from build123d import *

# Parameters (mm, degrees)
SKETCH1_W                      = 85
SKETCH1_H                      = 90
BOSS_EXTRUDE1_BASE_DEPTH       = 3
BOSS_EXTRUDE4_SIDE_WALLS_DEPTH = 90
CUT_EXTRUDE2_GUIDE_HOLES_DEPTH = 133.830719339
SKETCH15_W                     = 85
SKETCH15_H                     = 20
BOSS_EXTRUDE9_REAR_WALL_DEPTH  = 3
BOSS_EXTRUDE1_START            = 3
SKETCH17_W                     = 85
SKETCH17_H                     = 3
BOSS_EXTRUDE1_REAR_WALL_DEPTH  = 12
SKETCH30_W                     = 85
SKETCH30_H                     = 2
CUT_EXTRUDE1_REAR_WALL_DEPTH   = 10
BOSS_EXTRUDE2_START            = 25
SKETCH20_W                     = 3
SKETCH20_H                     = 87
BOSS_EXTRUDE2_SIDE_WALL_DEPTH  = 10
CHAMFER1_SIDE_WALL_SIZE        = 3
BOSS_EXTRUDE5_SIDE_WALL_DEPTH  = 30
CHAMFER2_ROOF_SIZE             = 30
CHAMFER2_ROOF_SIZE_2           = 170.138454589
SKETCH28_W                     = 85
SKETCH28_H                     = 91.38839507
BOSS_EXTRUDE7_ROOF_DEPTH       = 3
SKETCH29_W                     = 8.082998623
SKETCH29_H                     = 55.59785115
CUT_EXTRUDE1_CLEAN_UP_DEPTH    = 142.848358117
SKETCH31_W                     = 95
SKETCH31_H                     = 40
CUT_EXTRUDE2_CLEAN_UP_DEPTH    = 139.209678755


# Some blends are built 0.0001 mm under size
with BuildPart() as part:
    # Sketch1 → Boss-Extrude1 (Base) (new body)
    with BuildSketch(Plane(origin=(0, 0, 0), x_dir=(1, 0, 0), z_dir=(0, 1, 0))):
        with Locations((42.5, 45)):
            Rectangle(SKETCH1_W, SKETCH1_H)
    extrude(amount=BOSS_EXTRUDE1_BASE_DEPTH)

    # Sketch5 → Boss-Extrude4 (Side Walls) (add, through all)
    with BuildSketch(Plane.XY):
        Polygon((-5, 28.390936655), (0, 38), (0, 0), (-5, 9.609063345), align=None)
        Polygon((90, 9.609063345), (90, 28.390936655), (85, 38), (85, 0), align=None)
    extrude(amount=-BOSS_EXTRUDE4_SIDE_WALLS_DEPTH)

    # Sketch4 → Cut-Extrude2 (Guide Holes) (cut, through all)
    with BuildSketch(Plane.XY):
        Polygon((-3, 23), (0, 26), (0, 23), align=None)
        Polygon((85, 23), (88, 23), (85, 26), align=None)
    extrude(amount=-CUT_EXTRUDE2_GUIDE_HOLES_DEPTH, mode=Mode.SUBTRACT)

    # Sketch15 → Boss-Extrude9 (Rear Wall) (add)
    with BuildSketch(Plane.XY):
        with Locations((42.5, 13)):
            Rectangle(SKETCH15_W, SKETCH15_H)
    extrude(amount=-BOSS_EXTRUDE9_REAR_WALL_DEPTH)

    # Sketch17 → Boss-Extrude1 (Rear Wall) (add)
    with BuildSketch(Plane(origin=(0, 23, 0), x_dir=(1, 0, 0), z_dir=(0, 1, 0)).offset(BOSS_EXTRUDE1_START)):
        with Locations((42.5, 1.5)):
            Rectangle(SKETCH17_W, SKETCH17_H)
    extrude(amount=BOSS_EXTRUDE1_REAR_WALL_DEPTH)

    # Sketch30 → Cut-Extrude1 (Rear Wall) (cut)
    with BuildSketch(Plane.XY):
        with Locations((42.5, 27)):
            Rectangle(SKETCH30_W, SKETCH30_H)
    extrude(amount=-CUT_EXTRUDE1_REAR_WALL_DEPTH, mode=Mode.SUBTRACT)

    # Sketch20 → Boss-Extrude2 (Side Wall) (add)
    with BuildSketch(Plane(origin=(0, 3, 0), x_dir=(1, 0, 0), z_dir=(0, 1, 0)).offset(BOSS_EXTRUDE2_START)):
        with Locations((1.5, 46.5)):
            Rectangle(SKETCH20_W, SKETCH20_H)
        with Locations((83.5, 46.5)):
            Rectangle(SKETCH20_W, SKETCH20_H)
    extrude(amount=BOSS_EXTRUDE2_SIDE_WALL_DEPTH)

    # Chamfer1 (Side Wall)
    chamfer1_side_wall_edges = [part.edges().sort_by_distance(p)[0] for p in [
        (82, 28, -46.5),
        (3, 28, -46.5),
    ]]
    chamfer(chamfer1_side_wall_edges, length=CHAMFER1_SIDE_WALL_SIZE - 0.0001)  # a hair under: the kernel refuses the full size

    # Sketch26 → Boss-Extrude5 (Side Wall) (add)
    with BuildSketch(Plane(origin=(0, 38, 0), x_dir=(1, 0, 0), z_dir=(0, 1, 0))):
        Polygon((0, 0), (0, 90), (3, 90), (3, 3), (82, 3), (82, 90), (85, 90), (85, 0), align=None)
    extrude(amount=BOSS_EXTRUDE5_SIDE_WALL_DEPTH)

    # Chamfer2 (Roof)
    # the kernel refuses this chamfer: 170.138454589, 30 mm, written as the material it takes off along each edge
    with BuildSketch(Plane(origin=(527.111375011, 68, 0), x_dir=(0, -0.9776715712462578, 0.21013876076743532), z_dir=(-1, 0, 0))) as chamfer2_roof_piece_1:
        Polygon((CHAMFER2_ROOF_SIZE * 0.977671571246, -CHAMFER2_ROOF_SIZE * 0.210138760767), (-CHAMFER2_ROOF_SIZE_2 * 0.210138760767, -CHAMFER2_ROOF_SIZE_2 * 0.977671571244), (0, 0), align=None)
    extrude(amount=969.222750023, mode=Mode.SUBTRACT)

    # Sketch28 → Boss-Extrude7 (Roof) (add)
    with BuildSketch(Plane(origin=(0, 36.854159795, 6.498382723), x_dir=(1, 0, 0), z_dir=(0, 0.9848077530122086, 0.17364817766692742))):
        with Locations((42.5, 52.292828286)):
            Rectangle(SKETCH28_W, SKETCH28_H)
    extrude(amount=-BOSS_EXTRUDE7_ROOF_DEPTH)

    # Sketch29 → Cut-Extrude1 (Clean up) (cut, through all)
    with BuildSketch(Plane(origin=(90, 0, 0), x_dir=(0, 0, -1), z_dir=(1, 0, 0))):
        with Locations((94.041499312, 27.798925575)):
            Rectangle(SKETCH29_W, SKETCH29_H)
    extrude(amount=-CUT_EXTRUDE1_CLEAN_UP_DEPTH, mode=Mode.SUBTRACT)

    # Sketch31 → Cut-Extrude2 (Clean Up) (cut, through all)
    with BuildSketch(Plane.XZ):
        with Locations((42.5, -70)):
            Rectangle(SKETCH31_W, SKETCH31_H)
    extrude(amount=-CUT_EXTRUDE2_CLEAN_UP_DEPTH, mode=Mode.SUBTRACT)


solid = part.part
Model file for the job. Use its own axes, mm. A direction names the side the tool comes from. Give positions to 0.01 mm unless a question says otherwise; leave off trailing zeros. Order: outer loops, then holes, each group sorted by start corner. A loop starts at its lowest first (then second) coordinate and runs counter-clockwise, first axis right, second up. Notation, with made-up numbers: (10, 20.25) - (56, 20.25) arc R18 ccw to (56, 31.25) - close; hole circle Ø5 at (71.5, 28). An arc over 180 degrees is marked (long way). Write item = value, one per line. Start each with the question number.
1. Cut at C-C, the plane y = 17.5. List the corners of the cut face in (x, z), and give its area (3 significant figures).
2. Drop flat-ended pins along their axis: P1, Ø1.5, axis at x = 73.5, z = -31, coming from the +Y side; P2, Ø4.5, axis at y = 42, z = -15.5, coming from the -X side; P3, Ø14, axis at y = 38, z = -29.5, coming from the -X side. Give the stop position or say it passes through.
3. Probe line 1 along X through (y, z) = (21, -11.5); line 2 along Z through (x, y) = (58.5, 19); line 3 along Y through (x, z) = (38.5, -40). List the from-to ranges inside material, lowest first.
4. Which spindle directions (+Z, -Z, +X, -X, +Y, -Y) get a long thin tool onto all of the face, cutting with end or side? Do faces 1 (the flat face through (0, 40, -36)), 2 (the flat face through (0, 27, -25)), 3 (the flat face through (85, 13, -26)). Say none if no direction does.
5. Cut at A-A, the plane x = 57.5. List the corners of the cut face in (y, z).
6. Two-plate mould, pull along X, no slides. Class faces 4 (the flat face through (43.095, 42.346, -24.65)), 5 (the flat face through (0, 13, -26)), 6 (the flat face through (87.465, 4.737, -24.65)): pulls with the +X half, pulls with the -X half, needs draft (parallel to the pull), parting line crosses it, or undercut.
Taken from the geometry:
q1.outline = (-5, -50) - (0, -50) - (0, -3) - (85, -3) - (85, -50) - (90, -50) - (90, 0) - (-5, 0) - close
q1.area = 755 mm²
q2.P1 = 43.6
q2.P2 = 0
q2.P3 = -3.64
q3.line_1 = -5 to 0, 85 to 90
q3.line_2 = -3 to 0
q3.line_3 = 0 to 3, 42.01 to 45.05
q4.face_1 = +Z, -Z, -X, +Y
q4.face_2 = +Z, -Z
q4.face_3 = -Z
q5.outline = (0, -50) - (3, -50) - (3, -3) - (23, -3) - (23, 0) - (0, 0) - close; (28, -3) - (35.48, -3) - (43.77, -50) - (46.82, -50) - (38, 0) - (28, 0) - close
q6.face_4 = needs draft
q6.face_5 = undercut
q6.face_6 = pulls with the +X half
